Check sheet for the drawn part. Datum: minimum x, y, z corner. Units: mm. Coordinates: 2 decimals unless noted, no trailing zeros. Loops run counter-clockwise (first coordinate to the right, second up) from the corner with the lowest first, then second, coordinate; pieces in that order, holes last.
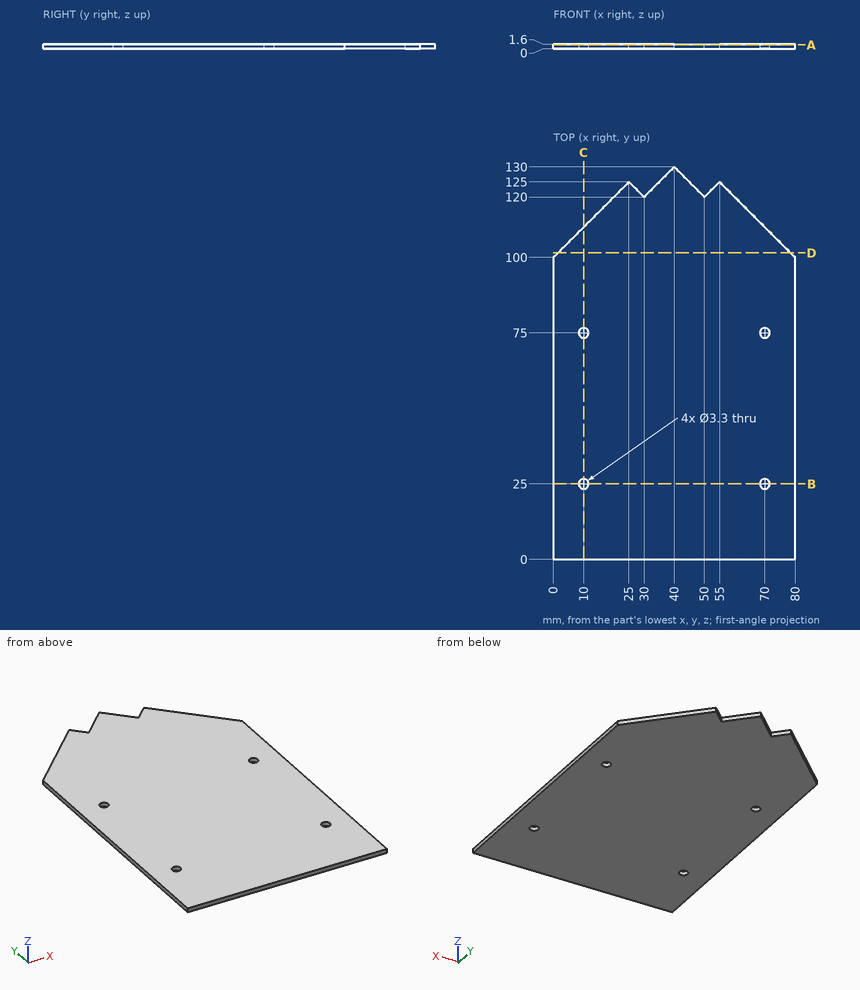
(1) Sectioned sample at C-C on x = 10. Record the cut outline in (y, z), and give its area (3 significant figures).
Findings:
outline: (0, 0) - (23.35, 0) - (23.35, 1.6) - (0, 1.6) - close; (26.65, 0) - (73.35, 0) - (73.35, 1.6) - (26.65, 1.6) - close; (76.65, 0) - (110, 0) - (110, 1.6) - (76.65, 1.6) - close
area: 165 mm2
(2) Sectioned sample at B-B on y = 25. Record the cut outline in (x, z).
Findings:
outline: (0, 0) - (8.35, 0) - (8.35, 1.6) - (0, 1.6) - close; (11.65, 0) - (68.35, 0) - (68.35, 1.6) - (11.65, 1.6) - close; (71.65, 0) - (80, 0) - (80, 1.6) - (71.65, 1.6) - close
(3) Sectioned sample at A-A on z = 1.35. Record the cut outline in (x, y).
Findings:
outline: (0, 0) - (80, 0) - (80, 100) - (55, 125) - (50, 120) - (40, 130) - (30, 120) - (25, 125) - (0, 100) - close; hole circle Ø3.3 at (10, 25); hole circle Ø3.3 at (10, 75); hole circle Ø3.3 at (70, 25); hole circle Ø3.3 at (70, 75)
(4) Scan lines: L1, parallel to X at y = 25, z = 0.8; L2, parallel to Y at x = 11.5, z = 0.95; L3, parallel to Y at x = 9, z = 0.75. Record each from-to range of solid material in increasing order.
Findings:
L1: x = 0 to 8.35, 11.65 to 68.35, 71.65 to 80
L2: y = 0 to 24.31, 25.69 to 74.31, 75.69 to 111.5
L3: y = 0 to 23.69, 26.31 to 73.69, 76.31 to 109
(5) Sectioned sample at D-D on y = 101.5. Record the cut outline in (x, z), and give its area (3 significant figures).
Findings:
outline: (1.5, 0) - (78.5, 0) - (78.5, 1.6) - (1.5, 1.6) - close
area: 123 mm2
